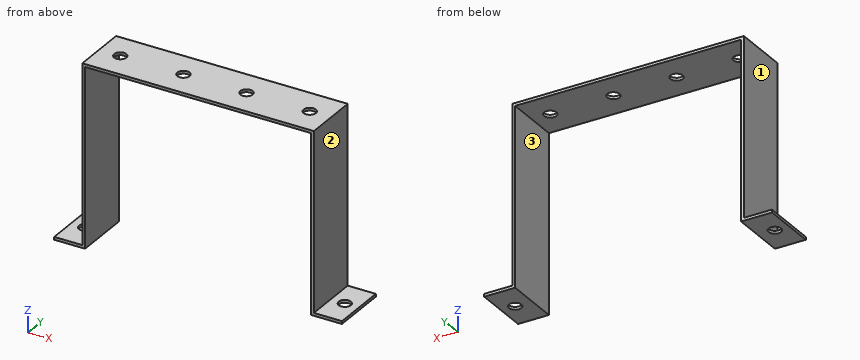
from build123d import *

# Parameters (mm, degrees)
F1_DEPTH   = 20
F5_D       = 8.8
F5_ON_F2_D = 8.8
F5_ON_F4_D = 8.8


with BuildPart() as f1:
    # F0 (on Front) → F1 (new body, symmetric)
    with BuildSketch(Plane.XZ):
        Polygon((74.3795982003, 82.5967788231), (-90.6204017997, 82.5967788231), (-90.6204017997, -44.3232211769), (-110.6204017997, -44.3232211769), (-110.6204017997, -46.3232211769), (-88.6204017997, -46.3232211769), (-88.6204017997, 80.5967788231), (-8.1204017997, 80.5967788231), (72.3795982003, 80.5967788231), (72.3795982003, -46.3232211769), (94.3795982003, -46.3232211769), (94.3795982003, -44.3232211769), (74.3795982003, -44.3232211769), align=None)
    extrude(amount=F1_DEPTH, both=True)

    # F5 (through all)
    with Locations(Plane.XY.offset(82.5967788231)):
        with Locations((-75.6204017997, 0), (-30.6204017997, 0), (14.3795982003, 0), (59.3795982003, 0)):
            Hole(F5_D / 2)

    # F5 on F2 (through all)
    with Locations(Plane.XY.offset(-44.3232211769)):
        with Locations((-100.6204017997, 0)):
            Hole(F5_ON_F2_D / 2)

    # F5 on F4 (through all)
    with Locations(Plane.XY.offset(-44.3232211769)):
        with Locations((84.3795982003, 0)):
            Hole(F5_ON_F4_D / 2)


solid = f1.part
Verification items for the finished model (mm, model axes). Face numbers are marked on the shaded views. A direction names the side the tool comes from. Coordinates: 2 decimals unless noted, no trailing zeros. Loops run counter-clockwise (first coordinate to the right, second up) from the corner with the lowest first, then second, coordinate; pieces in that order, holes last. Notation, with made-up numbers: (68, 77.25) -> (88, 77.25) arc R30 cw to (88, 100.25) -> close; hole circle Ø2 at (32.5, 83.5). An arc over 180 degrees is marked (long way). Answer as a JSON object with one key per item and string values. Group by question number.
Item 1: Sectioned sample at C-C on x = -63.5. Record the boundary of the cut face in (y, z).
Item 2: Sectioned sample at A-A on z = -12. Record the boundary of the cut face in (x, y).
Item 3: Depth check by flat-ended pin: pin 1 (16 mm diameter, centred on x = -101.5, y = -7.5, fed in from +Z); pin 2 (20 mm diameter, centred on y = -4, z = 25, fed in from -X); pin 3 (12 mm diameter, centred on y = 9.5, z = 13.5, fed in from +X). Enter the tip coordinate at first touch or a pass-through.
Item 4: Sectioned sample at B-B on y = 7.5. Record the boundary of the cut face in (x, z), plus the area to 3 significant figures.
Item 5: Tool access check on the marked faces 1, 2 and 3. Record the directions out of +Z, -Z, +X, -X, +Y, -Y that give a thin tool (end or side, any length) a straight path to the whole face; none if there is none.
Item 6: Scan lines: probe 1 along X at (y, z) = (-16, 7); probe 2 along Z at (x, y) = (32, 1); probe 3 along Z at (x, y) = (-95, 11). Record each from-to range of solid material in increasing order.
Evaluation:
{
 "1": {"outline": "(-20, 80.6) -> (20, 80.6) -> (20, 82.6) -> (-20, 82.6) -> close"},
 "2": {"outline": "(-90.62, -20) -> (-88.62, -20) -> (-88.62, 20) -> (-90.62, 20) -> close; (72.38, -20) -> (74.38, -20) -> (74.38, 20) -> (72.38, 20) -> close"},
 "3": {"pin 1": "stops at z = -44.32", "pin 2": "stops at x = -90.62", "pin 3": "stops at x = 74.38"},
 "4": {"outline": "(-110.62, -46.32) -> (-88.62, -46.32) -> (-88.62, 80.6) -> (72.38, 80.6) -> (72.38, -46.32) -> (94.38, -46.32) -> (94.38, -44.32) -> (74.38, -44.32) -> (74.38, 82.6) -> (-90.62, 82.6) -> (-90.62, -44.32) -> (-110.62, -44.32) -> close", "area": "918 mm²"},
 "5": {"face 1": "+Z, -X, +Y, -Y", "face 2": "+Z, +X, +Y, -Y", "face 3": "-Z, +Y, -Y"},
 "6": {"probe 1": "x = -90.62 to -88.62, 72.38 to 74.38", "probe 2": "z = 80.6 to 82.6", "probe 3": "z = -46.32 to -44.32"}
}
